Input: dimensioned drawing with shaded views. Units: mm. Origin: part minimum x, y, z. A direction names the side the tool comes from. Give positions to 0.01 mm unless a question says otherwise; leave off trailing zeros. Loops run counter-clockwise (first coordinate to the right, second up) from the corner with the lowest first, then second, coordinate; pieces in that order, holes last.
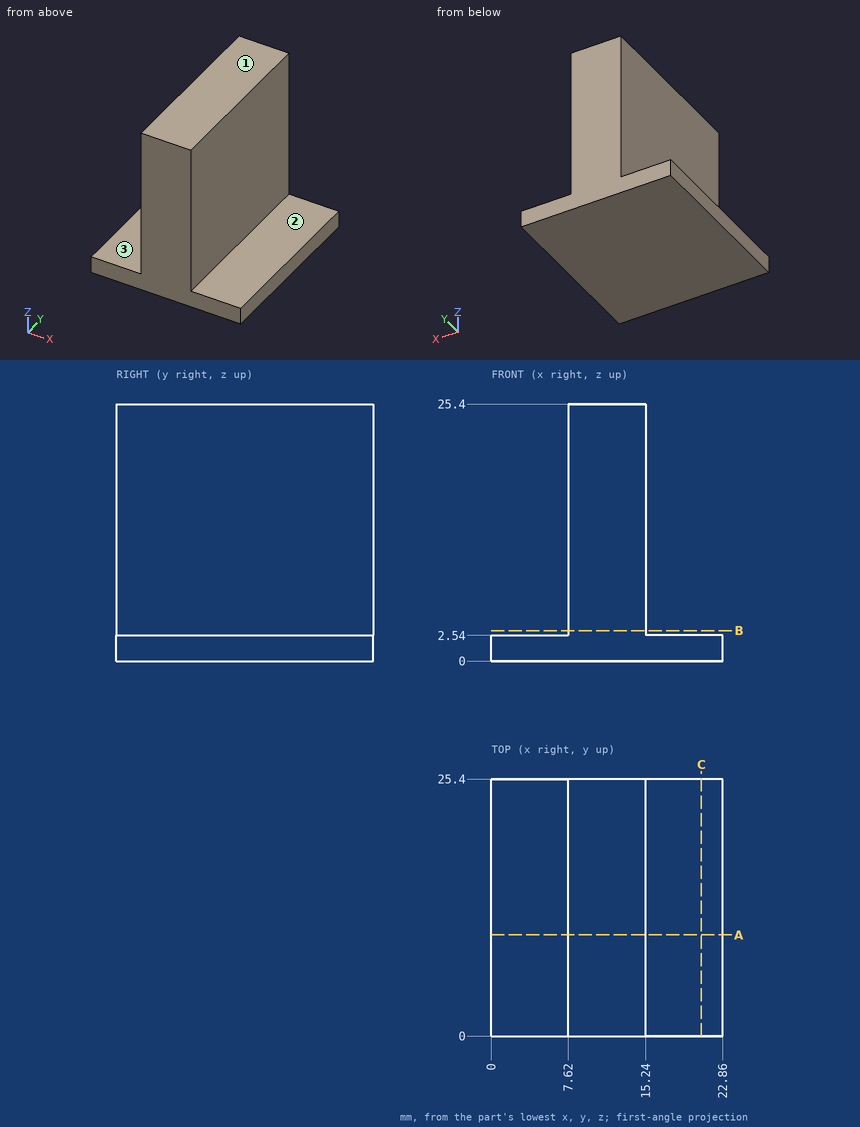
(1) Reachability of the marked faces 1, 2 and 3 from +Z, -Z, +X, -X, +Y, -Y: full face, straight path, thin tool, end or side. Return the list, or none.
A:
face 1: +Z, +X, -X, +Y, -Y
face 2: +Z, +X, +Y, -Y
face 3: +Z, -X, +Y, -Y
(2) Section C-C, the plane x = 20.75. Return the cut outline in (y, z), then the cut area to 3 significant figures.
A:
outline: (0, 0) - (25.4, 0) - (25.4, 2.54) - (0, 2.54) - close
area: 64.5 mm2
(3) Ray query, line 1 along X through (y, z) = (13, 18.75); line 2 along Z through (x, y) = (5.5, 8.5). Return the intervals inside material, ascending.
A:
line 1: x = 7.62 to 15.24
line 2: z = 0 to 2.54
(4) Section B-B, the plane z = 3. Return the cut outline in (x, y).
A:
outline: (7.62, 0) - (15.24, 0) - (15.24, 25.4) - (7.62, 25.4) - close
(5) Section A-A, the plane y = 10. Return the cut outline in (x, z), then the cut area to 3 significant figures.
A:
outline: (0, 0) - (22.86, 0) - (22.86, 2.54) - (15.24, 2.54) - (15.24, 25.4) - (7.62, 25.4) - (7.62, 2.54) - (0, 2.54) - close
area: 232 mm2
(6) First-contact query: pin 1 (3 mm diameter, centred on x = 6.5, z = 3.5, fed in from -Y); pin 2 (5 mm diameter, centred on y = 8.5, z = 8.5, fed in from +X); pin 3 (4 mm diameter, centred on x = 18, y = 11.5, fed in from +Z); pin 4 (11.5 mm diameter, centred on y = 11, z = 15.5, fed in from -X). Flat tips, straight axial feed; report the tip coordinate or a pass-through.
A:
pin 1: stops at y = 0
pin 2: stops at x = 15.24
pin 3: stops at z = 2.54
pin 4: stops at x = 7.62
